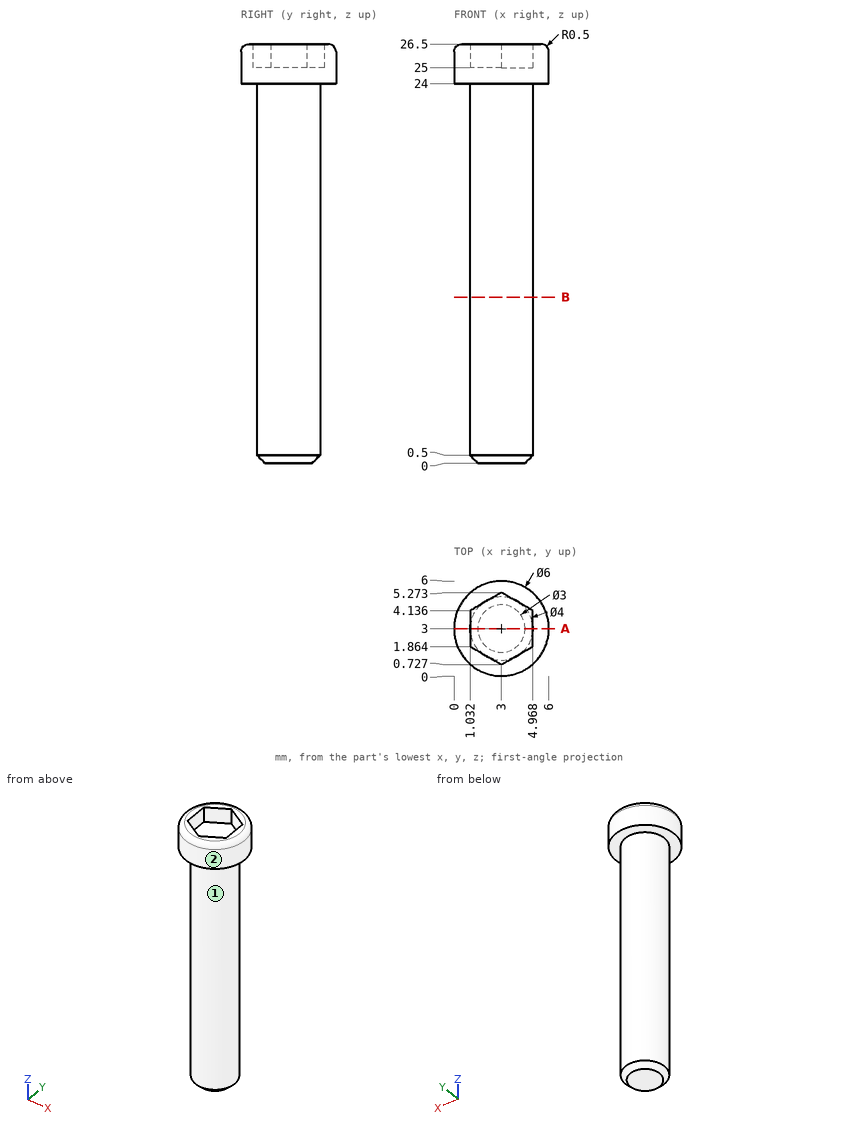
Print and shaded views of the part. All mm, measured from the part's lowest x, y and z. A direction names the side the tool comes from. Give positions to 0.01 mm unless a question says otherwise; leave off trailing zeros. Write each loop counter-clockwise with the first axis right and the second up, starting at its lowest first coordinate (ties: lowest second). Pieces come first, ordered by that corner, then holes. Notation, with made-up numbers: M 29,-13.5 L 67,-13.5 A18 ccw 67,-0.5 Z; hole C 44.25,47.5 d4. An arc over 180 degrees is marked long. Use a Markdown table: item, result.
1) Drill centre lines: line 1 (Z direction, x = 1.85, y = 0.95); line 2 (Y direction, x = 2.9, z = 19.75); line 3 (Z direction, x = 2.15, y = 3.3). Where is each one in solid material? Low to high. Write a range as from..to.
Responses:
| item | result |
|---|---|
| line 1 | z = 24..26.5 |
| line 2 | y = 1..5 |
| line 3 | z = 0..25 |
2) Cut at B-B (z = 10.5). List the corners of the cut face in (x, y).
Responses:
| item | result |
|---|---|
| outline | C 3,3 d4 |
3) Pin check, flat tips, straight feed: pin 1 (2 mm diameter, centred on x = 5, z = 15.5, fed in from +Y); pin 2 (2 mm diameter, centred on y = 1, z = 14.5, fed in from -X); pin 3 (2 mm diameter, centred on x = 1.5, z = 21.5, fed in from +Y). Stop position of each tip, or through.
Responses:
| item | result |
|---|---|
| pin 1 | stops at y = 4.73 |
| pin 2 | stops at x = 1.27 |
| pin 3 | stops at y = 4.94 |
4) Cut at A-A (y = 3). List the corners of the cut face in (x, z), and give its area (3 significant figures).
Responses:
| item | result |
|---|---|
| outline | M 0,24 L 1,24 L 1,0.5 L 1.5,0 L 4.5,0 L 5,0.5 L 5,24 L 6,24 L 6,26 A0.5 ccw 5.5,26.5 L 4.97,26.5 L 4.97,25 L 1.03,25 L 1.03,26.5 L 0.5,26.5 A0.5 ccw 0,26 Z |
| area | 105 mm2 |
5) Tool access for the marked faces 1 and 2: list every direction of +Z, -Z, +X, -X, +Y, -Y with a clear straight run to the whole face (end or side of a thin tool).
Responses:
| item | result |
|---|---|
| face 1 | -Z |
| face 2 | +Z, -Z |
